Can you work these out from the drawing? Everything is in mm from the part's minimum corner. A direction names the side the tool comes from. Coordinates: 2 decimals unless noted, no trailing zeros. Loops run counter-clockwise (first coordinate to the right, second up) from the corner with the lowest first, then second, coordinate; pieces in that order, holes last. Notation, with made-up numbers: (24, -21) -> (72, -21) arc R25 ccw to (72, 5) -> close; hole circle Ø7 at (-35, 85). An arc over 180 degrees is marked (long way). Use one line per item in the form item = value. Start each with the question number.
(1) Imagine slicing it at B-B (z = 6). List the corners of the cut face in (x, y) for me.
(2) I need wall thicknesses on line 1 (X direction, y = 2.25, z = 6); line 2 (Z direction, x = 3.75, y = 1.5). Which ranges of each line are inside material? Lowest first, please. Write a range as [from, to].
(3) Imagine slicing it at A-A (x = 6). List the corners of the cut face in (y, z) for me.
(4) Thinking about a two-plate mould opening in Z: for the marked faces 3, 4 and 5, which applies, released by +Z, released by -Z, zero draft, split by the parting line, or undercut?
(5) Imagine slicing it at C-C (y = 8.5). List the corners of the cut face in (x, z) for me, plus the area to 3 significant figures.
(6) I'm going to push flat-ended pins straight in: pin 1 (1 mm diameter, centred on y = 6, z = 8.5, fed in from -X); pin 2 (5 mm diameter, centred on x = 3.5, y = 6, fed in from +Z); pin 3 (2 mm diameter, centred on x = 3, z = 10.5, fed in from +Y). Where does each tip first touch, or does it pass through?
(7) On a 3-axis mill with a long thin cutter (end or side, diameter ignored), from which of +Z, -Z, +X, -X, +Y, -Y can I reach the whole of each face in a straight line? I mean the marked faces 1 and 2. Say none if no direction works.
(8) Imagine slicing it at D-D (x = 2.5). List the corners of the cut face in (y, z) for me, plus the area to 3 significant figures.
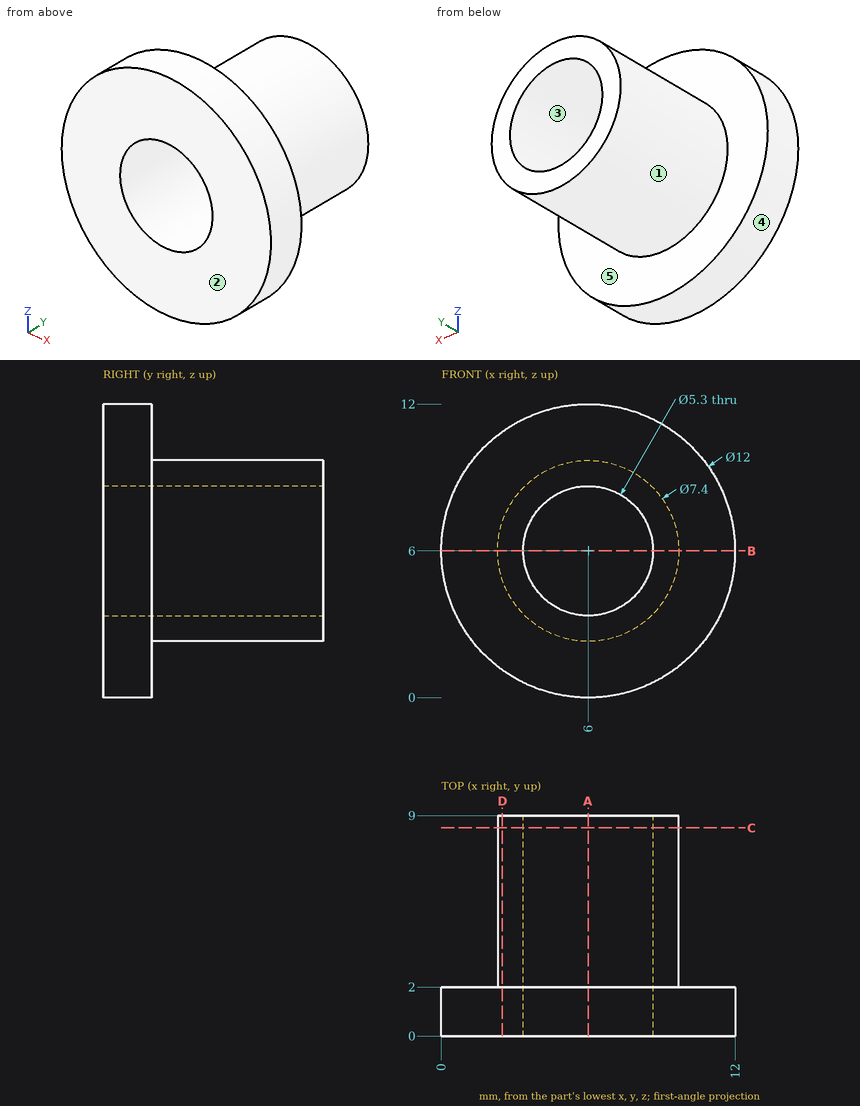
Worked out:
q1.outline = (0, 0) -> (3.35, 0) -> (3.35, 9) -> (2.3, 9) -> (2.3, 2) -> (0, 2) -> close; (8.65, 0) -> (12, 0) -> (12, 2) -> (9.7, 2) -> (9.7, 9) -> (8.65, 9) -> close
q2.line_1 = [2.3, 3.35], [8.65, 9.7]
q2.line_2 = [0.44, 4.6], [7.4, 11.56]
q3.outline = (0, 0) -> (2, 0) -> (2, 2.3) -> (9, 2.3) -> (9, 3.35) -> (0, 3.35) -> close; (0, 8.65) -> (9, 8.65) -> (9, 9.7) -> (2, 9.7) -> (2, 12) -> (0, 12) -> close
q4.face_3 = undercut
q4.face_4 = split by the parting line
q4.face_5 = zero draft
q5.outline = circle Ø7.4 at (6, 6); hole circle Ø5.3 at (6, 6)
q5.area = 20.9 mm2
q6.pin_1 = 2.89
q6.pin_2 = 9.7
q6.pin_3 = 2
q7.face_1 = +Y
q7.face_2 = +Z, -Z, +X, -X, -Y
q8.outline = (0, 1.13) -> (2, 1.13) -> (2, 4.8) -> (9, 4.8) -> (9, 7.2) -> (2, 7.2) -> (2, 10.87) -> (0, 10.87) -> close
q8.area = 36.3 mm2
